```python
from build123d import *

# Parameters (mm, degrees)
SKETCH_1_W          = 8.24
SKETCH_1_H          = 5.3
EXTRUDE_1_DEPTH     = 6.4
SKETCH_2_W          = 7.44
SKETCH_2_H          = 4.5
SKETCH_2_R          = 0.4
CUT_EXTRUDE_1_DEPTH = 5
SKETCH_3_W          = 9.698331409
SKETCH_3_H          = 0.501475964
CUT_EXTRUDE_2_DEPTH = 5
SKETCH_4_R          = 0.4
EXTRUDE_2_DEPTH     = 8


with BuildPart() as part:
    # Эскиз1 → Вытянуть1 (new body)
    with BuildSketch(Plane.XY):
        Rectangle(SKETCH_1_W, SKETCH_1_H)
    extrude(amount=EXTRUDE_1_DEPTH)

    # Эскиз2 → Вырез-Вытянуть1 (cut)
    with BuildSketch(Plane.XY.offset(6.4)):
        Rectangle(SKETCH_2_W, SKETCH_2_H)
        with Locations((-2.54, 0)):
            Circle(SKETCH_2_R, mode=Mode.SUBTRACT)
        with Locations((2.54, 0)):
            Circle(SKETCH_2_R, mode=Mode.SUBTRACT)
        with Locations((-0.030392483, 0)):
            Circle(SKETCH_2_R, mode=Mode.SUBTRACT)
    extrude(amount=-CUT_EXTRUDE_1_DEPTH, mode=Mode.SUBTRACT)

    # Эскиз3 → Вырез-Вытянуть2 (cut)
    with BuildSketch(Plane.XY.offset(6.4)):
        with Locations((-0.050465246, -2.002104797)):
            Rectangle(SKETCH_3_W, SKETCH_3_H)
    extrude(amount=-CUT_EXTRUDE_2_DEPTH, mode=Mode.SUBTRACT)

    # Эскиз4 → Вытянуть2 (add)
    with BuildSketch(Plane.XY.offset(6.4)):
        with Locations((-2.54, 0)):
            Circle(SKETCH_4_R)
        with Locations((2.54, 0)):
            Circle(SKETCH_4_R)
        with Locations((-0.030392483, 0)):
            Circle(SKETCH_4_R)
    extrude(amount=-EXTRUDE_2_DEPTH)


solid = part.part
```
Could you check a few things on this model? Use its own coordinates, in mm. A direction names the side the tool comes from. Round coordinates to 2 decimals unless told otherwise and drop trailing zeros. Loops run counter-clockwise (first coordinate to the right, second up) from the corner with the lowest first, then second, coordinate; pieces in that order, holes last. Notation, with made-up numbers: (-7, 43) -> (36, 43) arc R24 cw to (36, 66) -> close; hole circle Ø9 at (54.5, 69). An arc over 180 degrees is marked (long way). Put each result on its own line as item: value.
Q1. I want a section at D-D on y = 2. Write out the boundary of the cut face in (x, z).
Checks:
outline: (-4.12, 0) -> (4.12, 0) -> (4.12, 6.4) -> (3.72, 6.4) -> (3.72, 1.4) -> (-3.72, 1.4) -> (-3.72, 6.4) -> (-4.12, 6.4) -> close
Q2. Thinking about a two-plate mould opening in Y: for faces 4 (the flat face through (0, -2.65, 3)), 5 (the flat face through (3.72, 0, 4)), 6 (the flat face through (-4.12, 0, 3)), which applies, pulls with the +Y half, pulls with the -Y half, needs draft (parallel to the pull), parting line crosses it, or undercut?
Checks:
face 4: pulls with the -Y half
face 5: undercut
face 6: needs draft
Q3. I want a section at C-C on x = 2.54. Write out the boundary of the cut face in (y, z).
Checks:
outline: (-2.65, 0) -> (-0.4, 0) -> (-0.4, -1.6) -> (0.4, -1.6) -> (0.4, 0) -> (2.65, 0) -> (2.65, 6.4) -> (2.25, 6.4) -> (2.25, 1.4) -> (0.4, 1.4) -> (0.4, 6.4) -> (-0.4, 6.4) -> (-0.4, 1.4) -> (-2.25, 1.4) -> (-2.25, 6.4) -> (-2.65, 6.4) -> close
Q4. I want a section at A-A on z = 5.25. Write out the boundary of the cut face in (x, y).
Checks:
outline: (-4.12, -2.65) -> (4.12, -2.65) -> (4.12, -2.25) -> (-4.12, -2.25) -> close; (-4.12, -1.75) -> (-3.72, -1.75) -> (-3.72, 2.25) -> (3.72, 2.25) -> (3.72, -1.75) -> (4.12, -1.75) -> (4.12, 2.65) -> (-4.12, 2.65) -> close; circle Ø0.8 at (-2.54, 0); circle Ø0.8 at (-0.03, 0); circle Ø0.8 at (2.54, 0)
Q5. Please list where these lines run through material, in increasing order: line 1 (X direction, y = 0.05, z = 2.75); line 2 (Y direction, x = -1, z = 2.25); line 3 (X direction, y = -0.55, z = 2.75). Write a range as from..to.
Checks:
line 1: -4.12..-3.72, -2.94..-2.14, -0.43..0.37, 2.14..2.94, 3.72..4.12
line 2: -2.65..-2.25, 2.25..2.65
line 3: -4.12..-3.72, 3.72..4.12
Q6. Which directions (+Z, -Z, +X, -X, +Y, -Y) give clear straight access to the entire face, cutting with the end or side of a thin tool? Please do faces 1 (the flat face through (-3.72, 0, 4)), 2 (the flat face through (0, -2.253, 4)), 3 (the flat face through (0, 2.65, 3)).
Checks:
face 1: +Z
face 2: +Z, +X, -X
face 3: +Z, -Z, +X, -X, +Y
